from build123d import *

# Parameters (mm, degrees)
F0_R     = 1.1684
F1_DEPTH = 4.5085
F3_DEPTH = 4.953
F5_DEPTH = 4.4069
F6_R     = 0.254
F7_DEPTH = 3.81


with BuildPart() as f1:
    # F0 (on Top) → F1 (new body, symmetric)
    with BuildSketch(Plane.XY):
        with BuildLine():
            Line((17.2847, 3.937), (-17.2847, 3.937))
            ThreePointArc((-17.2847, 3.937), (-18.398252, 3.475752), (-18.8595, 2.3622))
            Line((-18.8595, 2.3622), (-18.8595, -2.3622))
            ThreePointArc((-18.8595, -2.3622), (-18.398252, -3.475752), (-17.2847, -3.937))
            Line((-17.2847, -3.937), (17.2847, -3.937))
            ThreePointArc((17.2847, -3.937), (18.398252, -3.475752), (18.8595, -2.3622))
            Line((18.8595, -2.3622), (18.8595, 2.3622))
            ThreePointArc((18.8595, 2.3622), (18.398252, 3.475752), (17.2847, 3.937))
        make_face()
        with Locations((-16.0655, 0)):
            Circle(F0_R, mode=Mode.SUBTRACT)
        with Locations((16.0655, 0)):
            Circle(F0_R, mode=Mode.SUBTRACT)
    extrude(amount=F1_DEPTH, both=True)

    # F2 (on face) → F3 (join)
    with BuildSketch(Plane.XY.offset(4.5085)):
        with BuildLine():
            Line((-12.59192, -3.2893), (12.593378, -3.2893))
            ThreePointArc((12.593378, -3.2893), (13.950271, -2.513771), (13.970729, -0.951022))
            Line((13.970729, -0.951022), (12.182639, 2.274778))
            ThreePointArc((12.182639, 2.274778), (11.604559, 2.868194), (10.805288, 3.0861))
            Line((10.805288, 3.0861), (-10.80383, 3.0861))
            ThreePointArc((-10.80383, 3.0861), (-11.603101, 2.868194), (-12.181181, 2.274778))
            Line((-12.181181, 2.274778), (-13.969271, -0.951022))
            ThreePointArc((-13.969271, -0.951022), (-13.948814, -2.513771), (-12.59192, -3.2893))
        make_face()
    extrude(amount=F3_DEPTH)

    # F4 (on face) → F5 (cut)
    with BuildSketch(Plane.XY.offset(9.4615)):
        with BuildLine():
            Line((10.618266, 2.7686), (-10.616808, 2.7686))
            ThreePointArc((-10.616808, 2.7686), (-11.41608, 2.550694), (-11.994159, 1.957278))
            Line((-11.994159, 1.957278), (-13.681127, -1.086092))
            ThreePointArc((-13.681127, -1.086092), (-13.664629, -2.346374), (-12.57036, -2.9718))
            Line((-12.57036, -2.9718), (12.571817, -2.9718))
            ThreePointArc((12.571817, -2.9718), (13.666086, -2.346374), (13.682584, -1.086092))
            Line((13.682584, -1.086092), (11.995617, 1.957278))
            ThreePointArc((11.995617, 1.957278), (11.417537, 2.550694), (10.618266, 2.7686))
        make_face()
    extrude(amount=-F5_DEPTH, mode=Mode.SUBTRACT)

    # F6 (on face) → F7 (join)
    with BuildSketch(Plane(origin=(0, 0, -4.5085), x_dir=(1, 0, 0), z_dir=(0, 0, -1))):
        with Locations((-10.4648, 1.905)):
            Circle(F6_R)
        with Locations((-8.5598, 1.905)):
            Circle(F6_R)
        with Locations((-6.6548, 1.905)):
            Circle(F6_R)
        with Locations((-4.7498, 1.905)):
            Circle(F6_R)
        with Locations((-2.8448, 1.905)):
            Circle(F6_R)
        with Locations((-0.9398, 1.905)):
            Circle(F6_R)
        with Locations((0.9652, 1.905)):
            Circle(F6_R)
        with Locations((2.8702, 1.905)):
            Circle(F6_R)
        with Locations((4.7752, 1.905)):
            Circle(F6_R)
        with Locations((6.6802, 1.905)):
            Circle(F6_R)
        with Locations((8.5852, 1.905)):
            Circle(F6_R)
        with Locations((10.4902, 1.905)):
            Circle(F6_R)
        with Locations((-11.4173, 0)):
            Circle(F6_R)
        with Locations((-9.5123, 0)):
            Circle(F6_R)
        with Locations((-7.6073, 0)):
            Circle(F6_R)
        with Locations((-5.7023, 0)):
            Circle(F6_R)
        with Locations((-3.7973, 0)):
            Circle(F6_R)
        with Locations((-1.8923, 0)):
            Circle(F6_R)
        with Locations((-10.4648, -1.905)):
            Circle(F6_R)
        with Locations((-8.5598, -1.905)):
            Circle(F6_R)
        with Locations((-6.6548, -1.905)):
            Circle(F6_R)
        with Locations((-4.7498, -1.905)):
            Circle(F6_R)
        with Locations((-2.8448, -1.905)):
            Circle(F6_R)
        with Locations((-0.9398, -1.905)):
            Circle(F6_R)
        with Locations((0.0127, 0)):
            Circle(F6_R)
        with Locations((1.9177, 0)):
            Circle(F6_R)
        with Locations((3.8227, 0)):
            Circle(F6_R)
        with Locations((5.7277, 0)):
            Circle(F6_R)
        with Locations((7.6327, 0)):
            Circle(F6_R)
        with Locations((9.5377, 0)):
            Circle(F6_R)
        with Locations((11.4427, 0)):
            Circle(F6_R)
        with Locations((0.9652, -1.905)):
            Circle(F6_R)
        with Locations((2.8702, -1.905)):
            Circle(F6_R)
        with Locations((4.7752, -1.905)):
            Circle(F6_R)
        with Locations((6.6802, -1.905)):
            Circle(F6_R)
        with Locations((8.5852, -1.905)):
            Circle(F6_R)
        with Locations((10.4902, -1.905)):
            Circle(F6_R)
    extrude(amount=F7_DEPTH)


solid = f1.part
Model file for the job. Use its own axes, mm. A direction names the side the tool comes from. Give positions to 0.01 mm unless a question says otherwise; leave off trailing zeros. Loops run counter-clockwise (first coordinate to the right, second up) from the corner with the lowest first, then second, coordinate; pieces in that order, holes last.
1) Wall check: line 1 (Y direction, x = -6, z = 6.5); line 2 (Z direction, x = -12, y = 1.75); line 3 (Z direction, x = 15, y = 1.5). Give the ranges that are in metal, low to high.
2) Pull direction X, two halves, no side cores. Call faces 1 (the flat face through (0, 3.937, 0)), 2 (the cylindrical face through (13.94, -2.53, 6.95)), 3 (the flat face through (-13.063, 0.684, 6.95)), 4 (the cylindrical face through (-11.406, 2.557, 7.289)): +X half, -X half, draft (parallel to the pull), parting line (faces both ways), or undercut.
3) Tool access for faces 5 (the cylindrical face through (-11.593, 2.874, 6.95)), 6 (the cylindrical face through (-13.96, -2.494, 6.95)), 7 (the flat face through (0, -2.972, 7)): list every direction of +Z, -Z, +X, -X, +Y, -Y with a clear straight run to the whole face (end or side of a thin tool).
4) Saw through at A-A (z = 7.5). Write the cut outline in (x, y).
5) Flat gauge pins, fed straight in: pin 1 Ø4 at (x, z) = (-6.5, 8) entering from -Y; pin 2 Ø3 at (x, y) = (-16.07, 0) entering from -Z; pin 3 Ø3 at (x, y) = (0.5, -1) entering from +Z. Where does each tip first touch, or does it go through?
Answer block:
1. line 1: y = -3.29 to -2.97, 2.77 to 3.09
1. line 2: z = -4.51 to 5.05
1. line 3: z = -4.51 to 4.51
2. face 1: draft
2. face 2: +X half
2. face 3: -X half
2. face 4: undercut
3. face 5: +Z, -X, +Y
3. face 6: +Z, -X
3. face 7: +Z
4. outline: (-13.97, -0.95) arc R1.57 ccw to (-12.59, -3.29) - (12.59, -3.29) arc R1.57 ccw to (13.97, -0.95) - (12.18, 2.27) arc R1.57 ccw to (10.81, 3.09) - (-10.8, 3.09) arc R1.57 ccw to (-12.18, 2.27) - close; hole (-13.68, -1.09) arc R1.27 ccw to (-12.57, -2.97) - (12.57, -2.97) arc R1.27 ccw to (13.68, -1.09) - (12, 1.96) arc R1.57 ccw to (10.62, 2.77) - (-10.62, 2.77) arc R1.57 ccw to (-11.99, 1.96) - close
5. pin 1: stops at y = -3.29
5. pin 2: stops at z = -4.51
5. pin 3: stops at z = 5.05
